Design review of the part built by this model. Coordinates are the model's own, in mm. Face numbers are marked on the shaded views. Give positions to 0.01 mm unless a question says otherwise; leave off trailing zeros. Order: outer loops, then holes, each group sorted by start corner. A loop starts at its lowest first (then second) coordinate and runs counter-clockwise, first axis right, second up. Notation, with made-up numbers: (-5.5, -23.75) -> (3.5, -23.75) arc R17 ccw to (3.5, -1.75) -> close; hole circle Ø3 at (40, 9). An arc over 180 degrees is marked (long way). One line per item, written item: value. Start each with the question number.
1) Consider section D-D (x = 1.35). State the section outline as (y, z) points.
2) For pin 1 (3.5 mm diameter, centred on y = 7.5, z = 0, fed in from -X); pin 2 (2.5 mm diameter, centred on y = 0, z = -7.5, fed in from -X); pin 3 (1.5 mm diameter, centred on x = 1.5, z = -1, fed in from +Y), all flat-tipped, find the tip position at first contact; note any pin that passes through.
3) Consider section B-B (z = 5). State the section outline as (x, y) points.
4) Wall thickness on line 1 along Y through (x, z) = (0.9, 1); line 2 along Z through (x, y) = (0.3, 12); line 3 along Y through (x, z) = (1.25, -7.5): over which ranges is each line inside the solid? List them lowest first. Write a range as from..to.
5) Consider section A-A (y = -50). State the section outline as (x, z) points, plus the area to 3 significant figures.
6) Consider section C-C (z = 0). State the section outline as (x, y) points, plus the area to 3 significant figures.
7) The part is to be moulded in two halves that separate along Z. For the marked faces 1, 2 and 3, say which applies: released by +Z, released by -Z, zero draft, split by the parting line, or undercut.
from build123d import *

# Parameters (mm, degrees)
CROQUIS1_R              = 3.5
CROQUIS1_R_2            = 1.5
SALIENTE_EXTRUIR1_DEPTH = 3


with BuildPart() as part:
    # Croquis1 → Saliente-Extruir1 (new body)
    with BuildSketch(Plane(origin=(0, 0, 0), x_dir=(0, 0, -1), z_dir=(1, 0, 0))):
        with BuildLine():
            ThreePointArc((14.657670874, 3.186327753), (-7.861609872, 12.774783372), (-9.449564448, -11.64928031))
            ThreePointArc((-9.449564448, -11.64928031), (-3.666028079, -29.56400504), (-9.338328875, -47.514260157))
            ThreePointArc((-9.338328875, -47.514260157), (-7.527733898, -54.313995983), (-0.71074339, -52.569489781))
            ThreePointArc((-0.71074339, -52.569489781), (13.908083657, -26.603024812), (14.657670874, 3.186327753))
        make_face()
        Circle(CROQUIS1_R, mode=Mode.SUBTRACT)
        with Locations((-5, -50)):
            Circle(CROQUIS1_R_2, mode=Mode.SUBTRACT)
        with Locations((-7.5, 0)):
            Circle(CROQUIS1_R_2, mode=Mode.SUBTRACT)
        with Locations((0, 7.5)):
            Circle(CROQUIS1_R_2, mode=Mode.SUBTRACT)
        with Locations((7.5, 0)):
            Circle(CROQUIS1_R_2, mode=Mode.SUBTRACT)
        with Locations((0, -7.5)):
            Circle(CROQUIS1_R_2, mode=Mode.SUBTRACT)
    extrude(amount=SALIENTE_EXTRUIR1_DEPTH)


solid = part.part
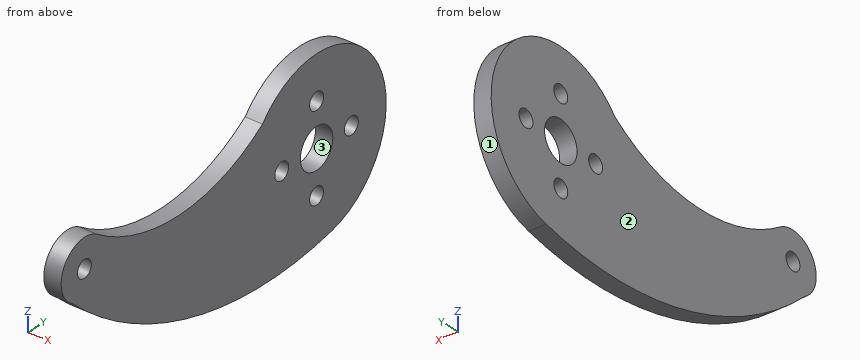
Checked values:
1. outline: (-52.57, 0.71) arc R61.72 ccw to (3.19, -14.66) arc R15 ccw (long way) to (-11.65, 9.45) arc R30.93 cw to (-47.51, 9.34) arc R5 ccw to start; hole circle Ø3 at (-50, 5); hole circle Ø3 at (-7.5, 0); hole circle Ø7 at (0, 0); hole circle Ø3 at (0, -7.5); hole circle Ø3 at (0, 7.5); hole circle Ø3 at (7.5, 0)
2. pin 1: stops at x = 0
2. pin 2: passes through
2. pin 3: stops at y = 15
3. outline: (0, -55) -> (3, -55) -> (3, -51.5) -> (0, -51.5) -> close; (0, -48.5) -> (3, -48.5) -> (3, -38.65) -> (0, -38.65) -> close; (0, -20.67) -> (3, -20.67) -> (3, 14.14) -> (0, 14.14) -> close
4. line 1: y = -53..-8.62, -6.38..-3.35, 3.35..6.38, 8.62..14.97
4. line 2: z = -9..9
4. line 3: y = -41.67..-1.5, 1.5..12.99
5. outline: (0, -1.58) -> (3, -1.58) -> (3, 3.5) -> (0, 3.5) -> close; (0, 6.5) -> (3, 6.5) -> (3, 10) -> (0, 10) -> close
5. area: 25.7 mm^2
6. outline: (0, -51.8) -> (3, -51.8) -> (3, -9) -> (0, -9) -> close; (0, -6) -> (3, -6) -> (3, -3.5) -> (0, -3.5) -> close; (0, 3.5) -> (3, 3.5) -> (3, 6) -> (0, 6) -> close; (0, 9) -> (3, 9) -> (3, 15) -> (0, 15) -> close
6. area: 161 mm^2
7. face 1: split by the parting line
7. face 2: zero draft
7. face 3: undercut
